from build123d import *

# Parameters (mm, degrees)
BOSS_EXTRUDE1_DEPTH      = 5
SKETCH1_3_R              = 15
BOSS_EXTRUDE2_DEPTH      = 20
BOSS_EXTRUDE2_DEPTH_BACK = 5
SKETCH1_4_R              = 17.5
BOSS_EXTRUDE3_DEPTH      = 5
BOSS_EXTRUDE3_DEPTH_BACK = 5


with BuildPart() as part:
    # Sketch1 → Boss-Extrude1 (new body)
    with BuildSketch(Plane.XY):
        with BuildLine():
            Line((50, 15), (9.615384615, 23.076923077))
            ThreePointArc((9.615384615, 23.076923077), (20.801257358, 13.867504906), (25, 0))
            ThreePointArc((25, 0), (20.801257358, -13.867504906), (9.615384615, -23.076923077))
            Line((9.615384615, -23.076923077), (50, -15))
            ThreePointArc((50, -15), (35, 0), (50, 15))
        make_face()
    extrude(amount=-BOSS_EXTRUDE1_DEPTH)

    # Sketch1_3 → Boss-Extrude2 (add, two sides)
    with BuildSketch(Plane.XY) as boss_extrude2_sk:
        with Locations((50, 0)):
            Circle(SKETCH1_3_R)
    extrude(amount=BOSS_EXTRUDE2_DEPTH)
    extrude(boss_extrude2_sk.sketch, amount=-BOSS_EXTRUDE2_DEPTH_BACK)

    # Sketch1_4 → Boss-Extrude3 (add, two sides)
    with BuildSketch(Plane.XY) as boss_extrude3_sk:
        with BuildLine():
            Line((9.615384615, 23.076923077), (0, 25))
            ThreePointArc((0, 25), (-25, 0), (0, -25))
            Line((0, -25), (9.615384615, -23.076923077))
            ThreePointArc((9.615384615, -23.076923077), (20.801257358, -13.867504906), (25, 0))
            ThreePointArc((25, 0), (20.801257358, 13.867504906), (9.615384615, 23.076923077))
        make_face()
        Circle(SKETCH1_4_R, mode=Mode.SUBTRACT)
    extrude(amount=BOSS_EXTRUDE3_DEPTH)
    extrude(boss_extrude3_sk.sketch, amount=-BOSS_EXTRUDE3_DEPTH_BACK)


solid = part.part
Geometry: final body of the model. Coordinates: model frame, mm. A direction names the side the tool comes from. Coordinates: 2 decimals unless noted, no trailing zeros. Write each loop counter-clockwise with the first axis right and the second up, starting at its lowest first coordinate (ties: lowest second). Pieces come first, ordered by that corner, then holes. Notation, with made-up numbers: (-38.5, 16) - (-31.5, 16) arc R22 cw to (-31.5, 22) - close; hole circle Ø9 at (72.5, 17). An arc over 180 degrees is marked (long way). Return JSON: item names as keys, results as strings.
Item 1: Section query A-A (z = 1.25). Output: boundary loops of the cut face in (x, y).
Completed:
{"outline": "(0, -25) - (9.62, -23.08) arc R25 ccw to (9.62, 23.08) - (0, 25) arc R25 ccw to start; circle Ø30 at (50, 0); hole circle Ø35 at (0, 0)"}
Item 2: Reachability of faces 1 (the face through (20, 21, -2)), 2 (the face through (-17, -5, 5)), 3 (the face through (64.307, 4.506, 7.325)) from +Z, -Z, +X, -X, +Y, -Y: full face, straight path, thin tool, end or side. Return the list, or none.
Completed:
{"face 1": "+Z, -Z, +X, +Y", "face 2": "+Z, -X, +Y, -Y", "face 3": "+Z"}
Item 3: Pull-direction query (X, two-part tool) for faces 4 (the face through (19.09, -21.18, -2.15)), 5 (the face through (30, 0, 0)), 6 (the face through (19, 0, -5)); classes: +X half, -X half, draft (parallel to the pull), parting line (faces both ways), or undercut.
Completed:
{"face 4": "+X half", "face 5": "undercut", "face 6": "draft"}
Item 4: Line query: L1, parallel to Y at x = 0, z = 3.9; L2, parallel to X at y = 2, z = 0.5; L3, parallel to Z at x = -4.5, y = 20.5. Output: solid intervals per line, ascending.
Completed:
{"L1": "y = -25 to -17.5, 17.5 to 25", "L2": "x = -24.92 to -17.39, 17.39 to 24.92, 35.13 to 64.87", "L3": "z = -5 to 5"}
Item 5: Section query B-B (y = 3). Output: boundary loops of the cut face in (x, z), and give its area (3 significant figures).
Completed:
{"outline": "(-24.82, -5) - (-17.24, -5) - (-17.24, 5) - (-24.82, 5) - close; (17.24, -5) - (64.7, -5) - (64.7, 20) - (35.3, 20) - (35.3, 0) - (24.82, 0) - (24.82, 5) - (17.24, 5) - close", "area": "939 mm2"}
Item 6: Section query D-D (x = 48). Output: boundary loops of the cut face in (y, z), and give its area (3 significant figures).
Completed:
{"outline": "(-15.4, -5) - (15.4, -5) - (15.4, 0) - (14.87, 0) - (14.87, 20) - (-14.87, 20) - (-14.87, 0) - (-15.4, 0) - close", "area": "749 mm2"}
Item 7: Section query C-C (x = -15). Output: boundary loops of the cut face in (y, z), and give its area (3 significant figures).
Completed:
{"outline": "(-20, -5) - (-9.01, -5) - (-9.01, 5) - (-20, 5) - close; (9.01, -5) - (20, -5) - (20, 5) - (9.01, 5) - close", "area": "220 mm2"}
Item 8: Pin query (flat end, axial travel): pin 1 Ø6 at (x, z) = (41.5, 15) entering from +Y; pin 2 Ø5 at (y, z) = (-6, 13) entering from -X; pin 3 Ø3 at (x, y) = (39.5, 16) entering from +Z. Return the tip coordinate at first contact, or that it passes through.
Completed:
{"pin 1": "stops at y = 13.96", "pin 2": "stops at x = 35.41", "pin 3": "stops at z = 0"}
